```python
from build123d import *

# Parameters (mm, degrees)
SKETCH_1_W      = 15.5
SKETCH_1_H      = 5.1
EXTRUDE_1_DEPTH = 8.1
CHAMFER_1_SIZE  = 4
CHAMFER_2_SIZE  = 0.5
SKETCH_2_R      = 3.35
EXTRUDE_2_DEPTH = 7
SKETCH_3_R      = 3
EXTRUDE_3_DEPTH = 0.9
SKETCH_5_R      = 3.35
EXTRUDE_4_DEPTH = 20
CHAMFER_3_SIZE  = 1


with BuildPart() as part:
    # 草图1 → 凸台-拉伸1 (new body)
    with BuildSketch(Plane.XY):
        Rectangle(SKETCH_1_W, SKETCH_1_H)
    extrude(amount=EXTRUDE_1_DEPTH)

    # 倒角1
    chamfer_1_edges = [part.edges().sort_by_distance(p)[0] for p in [
        (-7.75, 2.55, 4.05),
        (7.75, 2.55, 4.05),
    ]]
    chamfer(chamfer_1_edges, length=CHAMFER_1_SIZE)

    # 倒角2
    chamfer_2_edges = [part.edges().sort_by_distance(p)[0] for p in [
        (0, 2.55, 0),
        (0, 2.55, 8.1),
        (-7.75, -2, 0),
        (-5.75, 0.55, 0),
        (5.75, 0.55, 0),
        (-7.75, -2, 8.1),
        (-5.75, 0.55, 8.1),
        (5.75, 0.55, 8.1),
        (7.75, -2, 8.1),
        (7.75, -2, 0),
    ]]
    chamfer(chamfer_2_edges, length=CHAMFER_2_SIZE)

    # 草图2 → 凸台-拉伸2 (add)
    with BuildSketch(Plane.XZ.offset(2.55)):
        with Locations(Location((0, 4.05, 0), (0, 0, 90))):
            Circle(SKETCH_2_R)
    extrude(amount=EXTRUDE_2_DEPTH)

    # 草图3 → 凸台-拉伸3 (add)
    with BuildSketch(Plane.XZ.offset(9.55)):
        with Locations(Location((0, 4.05, 0), (0, 0, 270))):
            Circle(SKETCH_3_R)
    extrude(amount=EXTRUDE_3_DEPTH)

    # 草图5 → 凸台-拉伸4 (add)
    with BuildSketch(Plane.XZ.offset(10.45)):
        with Locations(Location((0, 4.05, 0), (0, 0, 90))):
            Circle(SKETCH_5_R)
    extrude(amount=EXTRUDE_4_DEPTH)

    # 倒角3
    chamfer_3_edges = [part.edges().sort_by_distance(p)[0] for p in [
        (0, -30.45, 0.7),
    ]]
    chamfer(chamfer_3_edges, length=CHAMFER_3_SIZE)

    # 草图6 → 切除-旋转1 (revolve, cut)
    with BuildSketch(Plane(origin=(0, 0, 0), x_dir=(0, 0, -1), z_dir=(1, 0, 0)), mode=Mode.PRIVATE) as cut_revolve_1_sk:
        Polygon((-7.4, -22.455131571), (-7.4, -19.455131571), (-4.4, -22.455131571), align=None)
    revolve(cut_revolve_1_sk.sketch.rotate(Axis((0, -22.455131571, 7.4), (0, 0, -1)), 90), axis=Axis((0, -22.455131571, 7.4), (0, 0, -1)), mode=Mode.SUBTRACT)


solid = part.part
```
Source: CAD feature listing. Evaluate the final solid. Frame: model axes, mm. A direction names the side the tool comes from. Round coordinates to 2 decimals unless told otherwise and drop trailing zeros. Loops run counter-clockwise (first coordinate to the right, second up) from the corner with the lowest first, then second, coordinate; pieces in that order, holes last. Notation, with made-up numbers: (87, -12.75) - (137, -12.75) arc R22 ccw to (137, 19.25) - close; hole circle Ø9 at (38.5, 23). An arc over 180 degrees is marked (long way). Use CSV: the item, a comma, the result in double quotes.
Q1. Reachability of faces 1 (the cylindrical face through (-0.1, -19.8, 0.7)), 2 (the flat face through (-5.7, 0.6, 4)), 3 (the cylindrical face through (0.9, -9.99, 1.19)) from +Z, -Z, +X, -X, +Y, -Y: full face, straight path, thin tool, end or side. Return the list, or none.
Reported:
face 1,"-Y"
face 2,"+Z, -Z, -X, +Y"
face 3,"none"
Q2. Section query B-B, the plane y = -4.5. Output: boundary loops of the cut face in (x, z).
Reported:
outline,"circle Ø6.7 at (0, 4.05)"
Q3. Section query D-D, the plane x = 5. Output: boundary loops of the cut face in (y, z).
Reported:
outline,"(-2.55, 0) - (0.59, 0) - (1.3, 0.5) - (1.3, 7.6) - (0.59, 8.1) - (-2.55, 8.1) - close"
Q4. Pin query (flat end, axial travel): pin 1 Ø6 at (x, y) = (-0.5, -10.5) entering from +Z. Return the tip coordinate at first contact, or that it passes through.
Reported:
pin 1,"z = 7.4"
Q5. Section query A-A, the plane z = 4.05. Output: boundary loops of the cut face in (x, y), then the cut area to 3 significant figures.
Reported:
outline,"(-7.75, -2.55) - (-3.35, -2.55) - (-3.35, -9.55) - (-3, -9.55) - (-3, -10.45) - (-3.35, -10.45) - (-3.35, -29.45) - (-2.35, -30.45) - (2.35, -30.45) - (3.35, -29.45) - (3.35, -10.45) - (3, -10.45) - (3, -9.55) - (3.35, -9.55) - (3.35, -2.55) - (7.75, -2.55) - (7.75, -1.45) - (3.75, 2.55) - (-3.75, 2.55) - (-7.75, -1.45) - close"
area,"248 mm^2"
Q6. Section query C-C, the plane x = -5.75. Output: boundary loops of the cut face in (y, z).
Reported:
outline,"(-2.55, 0) - (-0.16, 0) - (0.55, 0.5) - (0.55, 7.6) - (-0.16, 8.1) - (-2.55, 8.1) - close"
Q7. Ray query, line 1 along Y through (x, z) = (-3.25, 6.5); line 2 along Y through (x, z) = (-2.75, 5.75); line 3 along X through (y, z) = (-25, 4.25). Return the intervals inside material, ascending.
Reported:
line 1,"-2.55 to 2.55"
line 2,"-29.57 to -10.45, -9.55 to 2.55"
line 3,"-3.34 to 3.34"
Q8. Mould query, pull axis X, two halves, no side actions, for faces 4 (the flat face through (3, -9.55, 3)), 5 (the flat face through (-5.599, 0.343, 7.854)), 6 (the cylindrical face through (1.283, -6.001, 7.145)), 7 (the conical face through (0.44, -22.27, 4.88)). Classes: pulls with the +X half, pulls with the -X half, needs draft (parallel to the pull), parting line crosses it, or undercut.
Reported:
face 4,"needs draft"
face 5,"pulls with the -X half"
face 6,"parting line crosses it"
face 7,"undercut"
